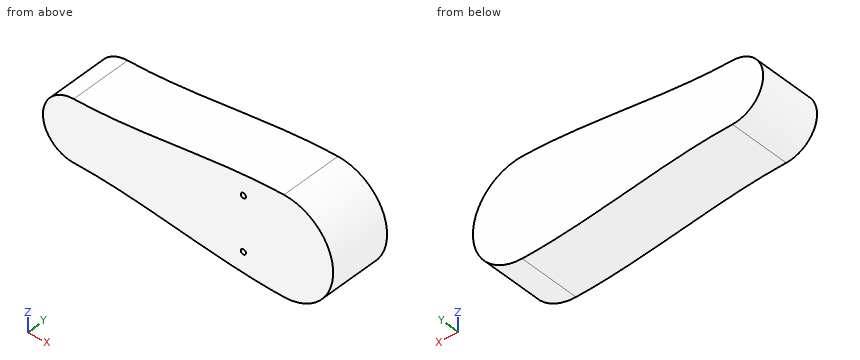
```python
from build123d import *

# Parameters (mm, degrees)
BOSS_EXTRUDE1_DEPTH   = 50
M5_TAPPED_HOLE1_D     = 4.2
M5_TAPPED_HOLE1_DEPTH = 14
M5_TAPPED_HOLE1_TIP   = 1.2618073


with BuildPart() as part:
    # Sketch1 → Boss-Extrude1 (new body)
    with BuildSketch(Plane(origin=(0, 0, 0), x_dir=(1, 0, 0), z_dir=(0, 1, 0))):
        with BuildLine():
            ThreePointArc((25, 50), (0, 25), (25, 0))
            add(Edge.make_bspline(
                [(25, 0), (82.580830765, 0), (138.63084141, -15), (195.775010008, -15)],
                knots=[0, 0, 0, 0, 1, 1, 1, 1], degree=3))
            ThreePointArc((195.775010008, -15), (235.775010008, 25), (195.775010008, 65))
            add(Edge.make_bspline(
                [(25, 50), (82.580830765, 50), (138.63084141, 65), (195.775010008, 65)],
                knots=[0, 0, 0, 0, 1, 1, 1, 1], degree=3))
        make_face()
    extrude(amount=BOSS_EXTRUDE1_DEPTH)

    # M5 Tapped Hole1
    with Locations(Plane(origin=(0, 0, 0), x_dir=(-1, 0, 0), z_dir=(0, -1, 0))):
        with Locations((-162.775010008, 3), (-162.775010008, 47)):
            Hole(M5_TAPPED_HOLE1_D / 2, depth=M5_TAPPED_HOLE1_DEPTH)
            with Locations((0, 0, -(M5_TAPPED_HOLE1_DEPTH + M5_TAPPED_HOLE1_TIP / 2))):  # 118° drill point
                Cone(0, M5_TAPPED_HOLE1_D / 2, M5_TAPPED_HOLE1_TIP, mode=Mode.SUBTRACT)


solid = part.part
```
The model under review builds one solid part; all positions refer to its coordinate system, in mm. Round coordinates to 2 decimals unless told otherwise and drop trailing zeros. One line per question, with ' | ' between items.
Item 1: Add section A-A, the plane y = 3.5. State how many separate pieces and enclosed holes the cut face has, then the cut area to 3 significant figures.
Resolved:
separate pieces: 1 | enclosed holes: 2 | area: 14,600 mm2
Item 2: For P1, Ø8, axis at y = 34, z = -52, coming from the -X side; P2, Ø10, axis at y = 23, z = -3, coming from the -X side; P3, Ø6.5, axis at x = 162.78, z = -3, coming from the -Y side; P4, Ø8, axis at y = 35.5, z = -1, coming from the -X side, all flat-tipped, find the tip position at first contact; note any pin that passes through.
Resolved:
P1: stops at x = 15.2 | P2: stops at x = 6.67 | P3: stops at y = 0 | P4: stops at x = 10
Item 3: To check wall thickness, follow probe 1 along X at (y, z) = (9.5, -47); probe 2 along Z at (x, y) = (24, 32); probe 3 along Z at (x, y) = (195.5, 45). State the ranges of each line that lie inside material, in increasing order.
Resolved:
probe 1: x = 13.13 to 160.68, 164.88 to 229.18 | probe 2: z = -49.98 to -0.02 | probe 3: z = -65 to 15
